```python
from build123d import *

# Parameters (mm, degrees)
SKETCH1_R           = 2
BOSS_EXTRUDE1_DEPTH = 8.89
CUT_EXTRUDE1_START  = -2.54
SKETCH2_R           = 2
SKETCH2_R_2         = 1.275
CUT_EXTRUDE1_DEPTH  = 2.54
FILLET2_R           = 0.508


with BuildPart() as part:
    # Sketch1 → Boss-Extrude1 (new body)
    with BuildSketch(Plane.XY):
        Circle(SKETCH1_R)
    extrude(amount=BOSS_EXTRUDE1_DEPTH)

    # Sketch2 → Cut-Extrude1 (cut)
    with BuildSketch(Plane.XY.offset(8.89).offset(CUT_EXTRUDE1_START)):
        Circle(SKETCH2_R)
        Circle(SKETCH2_R_2, mode=Mode.SUBTRACT)
    extrude(amount=CUT_EXTRUDE1_DEPTH, mode=Mode.SUBTRACT)

    # Fillet2
    fillet2_edges = [part.edges().sort_by_distance(p)[0] for p in [
        (-1.275, 0, 8.89),
    ]]
    fillet(fillet2_edges, radius=FILLET2_R)


solid = part.part
```
The listing builds one solid part. Answer for the finished solid, in the listing's coordinates (mm). A direction names the side the tool comes from. Coordinates: 2 decimals unless noted, no trailing zeros. Write each loop counter-clockwise with the first axis right and the second up, starting at its lowest first coordinate (ties: lowest second). Pieces come first, ordered by that corner, then holes. Notation, with made-up numbers: (84.5, 2.5) - (113.5, 2.5) arc R31 cw to (113.5, 38.5) - close; hole circle Ø7 at (-23.5, 89.5). An arc over 180 degrees is marked (long way). Return JSON: item names as keys, results as strings. Group by question number.
1. Straight lines are drawn through the part: L1, parallel to Z at x = 0.45, y = -1.3; L2, parallel to X at y = -1.75, z = 3.25; L3, parallel to Y at x = 0.75, z = 1.25. For each, find the intervals that lie inside material, in ascending order.
2. Given pin 1 (1 mm diameter, centred on x = -1, z = 7.5, fed in from -Y); pin 2 (2 mm diameter, centred on x = 1, z = 4, fed in from -Y); pin 3 (1.5 mm diameter, centred on y = -1, z = 7.5, fed in from -X), each flat-ended and moving along its own axis, determine where each tip first touches the part or whether it passes through.
3. A cutting plane is placed at A-A, the plane x = 0. Determine the outline of the cut face in (y, z) (3 decimals), plus the area to 3 significant figures.
4. A cutting plane is placed at D-D, the plane z = 0.75. Determine the outline of the cut face in (x, y), plus the area to 3 significant figures.
5. Which of the six approach directions +Z, -Z, +X, -X, +Y, -Y give full straight-line access (tool end or side, diameter ignored) to faces 1 (the cylindrical face through (0.59, -1.13, 7.35)), 2 (the cylindrical face through (0, -2, 3))?
6. A cutting plane is placed at C-C, the plane z = 7.25. Determine the outline of the cut face in (x, y) (3 decimals).
Ans:
{
 "1": {"L1": "0 to 6.35", "L2": "-0.97 to 0.97", "L3": "-1.85 to 1.85"},
 "2": {"pin 1": "y = -1.17", "pin 2": "y = -2", "pin 3": "x = -1.25"},
 "3": {"outline": "(-2, 0) - (2, 0) - (2, 6.35) - (1.275, 6.35) - (1.275, 8.382) arc R0.508 ccw to (0.767, 8.89) - (-0.767, 8.89) arc R0.508 ccw to (-1.275, 8.382) - (-1.275, 6.35) - (-2, 6.35) - close", "area": "31.8 mm²"},
 "4": {"outline": "circle Ø4 at (0, 0)", "area": "12.6 mm²"},
 "5": {"face 1": "+Z", "face 2": "+Z, -Z"},
 "6": {"outline": "circle Ø2.55 at (0, 0)"}
}
